Work out the finished part from the listing and answer in its coordinate system (mm). Round coordinates to 2 decimals unless told otherwise and drop trailing zeros. Order: outer loops, then holes, each group sorted by start corner. A loop starts at its lowest first (then second) coordinate and runs counter-clockwise, first axis right, second up. Notation, with made-up numbers: (-27, -32.5) - (-9, -32.5) arc R16 ccw to (-9, -3.5) - close; hole circle Ø3 at (49.5, 88.25). An arc over 180 degrees is marked (long way). Answer in a Markdown table with one row per item.
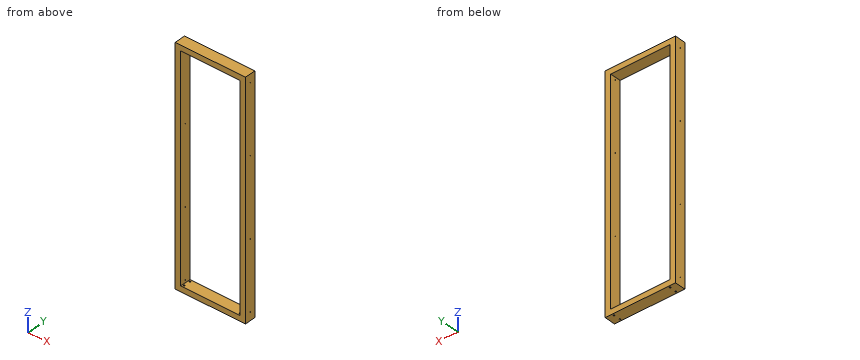
from build123d import *

# Parameters (mm, degrees)
F0_W     = 515
F0_H     = 1690
F0_W_2   = 435
F0_H_2   = 1610
F1_DEPTH = 80
F2_R     = 5
F3_DEPTH = 100
F4_R     = 2.5
F5_DEPTH = 1000


with BuildPart() as f1:
    # F0 (on Front) → F1 (new body)
    with BuildSketch(Plane.XZ):
        Rectangle(F0_W, F0_H)
        Rectangle(F0_W_2, F0_H_2, mode=Mode.SUBTRACT)
    extrude(amount=F1_DEPTH)

    # F2 (on face) → F3 (cut)
    with BuildSketch(Plane(origin=(0, 0, -845), x_dir=(1, 0, 0), z_dir=(0, 0, -1))):
        with Locations((-205, 65)):
            Circle(F2_R)
        with Locations((-205, 15)):
            Circle(F2_R)
        with Locations((205, 65)):
            Circle(F2_R)
        with Locations((205, 15)):
            Circle(F2_R)
    extrude(amount=-F3_DEPTH, mode=Mode.SUBTRACT)

    # F4 (on Right) → F5 (cut, symmetric)
    with BuildSketch(Plane.YZ):
        with Locations((-40, 285)):
            Circle(F4_R)
        with Locations((-40, 785)):
            Circle(F4_R)
        with Locations((-40, -285)):
            Circle(F4_R)
        with Locations((-40, -785)):
            Circle(F4_R)
    extrude(amount=F5_DEPTH, both=True, mode=Mode.SUBTRACT)


solid = f1.part
1) Find the intervals of material crossed by probe 1 along Z at (x, y) = (235, -40); probe 2 along Y at (x, z) = (205, -819); probe 3 along X at (y, z) = (-65, -830), in increasing order. Write a range as from..to.
Filled in:
| item | result |
|---|---|
| probe 1 | z = -845..-787.5, -782.5..-287.5, -282.5..282.5, 287.5..782.5, 787.5..845 |
| probe 2 | y = -80..-70, -60..-20, -10..0 |
| probe 3 | x = -257.5..-210, -200..200, 210..257.5 |
2) Find section A-A, the plane x = -12.5. Give the vertices of the cut face in (y, z).
Filled in:
| item | result |
|---|---|
| outline | (-80, -845) - (0, -845) - (0, -805) - (-80, -805) - close; (-80, 805) - (0, 805) - (0, 845) - (-80, 845) - close |
3) Find section B-B, the plane z = 302. Give the vertices of the cut face in (x, y).
Filled in:
| item | result |
|---|---|
| outline | (-257.5, -80) - (-217.5, -80) - (-217.5, 0) - (-257.5, 0) - close; (217.5, -80) - (257.5, -80) - (257.5, 0) - (217.5, 0) - close |
